Check sheet for the modelled part. Datum: model origin and axes. Units: mm. A direction names the side the tool comes from. Round coordinates to 2 decimals unless told otherwise and drop trailing zeros. Write each loop counter-clockwise with the first axis right and the second up, starting at its lowest first coordinate (ties: lowest second). Pieces come first, ordered by that corner, then holes. Notation, with made-up numbers: M 2,31 L 47,31 A27 ccw 47,47 Z; hole C 74,-23.75 d3. An arc over 180 degrees is marked long. One line per item, written item: value.
from build123d import *

# Parameters (mm, degrees)
F0_W     = 95.25
F0_H     = 304.8
F0_W_2   = 69.85
F0_H_2   = 292.1
F1_DEPTH = 69.85
F2_DEPTH = 6.35
F3_W     = 69.85
F3_H     = 76.2
F4_DEPTH = 6.35
F6_DEPTH = 450.85


with BuildPart() as f1:
    # F0 (on Top) → F1 (new body)
    with BuildSketch(Plane.XY):
        Rectangle(F0_W, F0_H)
        Rectangle(F0_W_2, F0_H_2, mode=Mode.SUBTRACT)
    extrude(amount=F1_DEPTH)

    # F0 (on Top) → F2 (join)
    with BuildSketch(Plane.XY):
        Rectangle(F0_W, F0_H)
        Rectangle(F0_W_2, F0_H_2, mode=Mode.SUBTRACT)
        Rectangle(F0_W_2, F0_H_2)
    extrude(amount=-F2_DEPTH)

    # F3 (on face) → F4 (cut)
    with BuildSketch(Plane(origin=(0, 0, -6.35), x_dir=(1, 0, 0), z_dir=(0, 0, -1))):
        with Locations((0, -107.95)):
            Rectangle(F3_W, F3_H)
    extrude(amount=-F4_DEPTH, mode=Mode.SUBTRACT)

    # F5 (on face) → F6 (join)
    with BuildSketch(Plane(origin=(0, 0, -6.35), x_dir=(1, 0, 0), z_dir=(0, 0, -1))):
        Polygon((-47.625, -152.4), (47.625, -152.4), (47.625, -95.25), (34.925, -95.25), (34.925, -146.05), (-34.925, -146.05), (-34.925, -95.25), (-47.625, -95.25), align=None)
    extrude(amount=F6_DEPTH)


solid = f1.part
Q1. Access from +Z, -Z, +X, -X, +Y, -Y to the whole of each face (thin tool, end or side, straight path). Record for faces 1 (the flat face through (34.925, 97, -75)), 2 (the flat face through (-41, 95.25, -229)), 3 (the flat face through (-1, -152.4, 32)).
Completed:
face 1: +Z
face 2: -Z, +X, -X, -Y
face 3: +Z, -Z, +X, -X, -Y
Q2. Sectioned sample at A-A on x = 9. Enter the section's corners in (y, z).
Completed:
outline: M -152.4,-6.35 L 69.85,-6.35 L 69.85,0 L -146.05,0 L -146.05,69.85 L -152.4,69.85 Z; M 146.05,-457.2 L 152.4,-457.2 L 152.4,69.85 L 146.05,69.85 Z
Q3. Depth check by flat-ended pin: P1, Ø3, axis at x = -22.5, y = -94, coming from the +Z side; P2, Ø4, axis at x = -41.5, z = -344, coming from the -Y side; P3, Ø2, axis at x = -19, y = 14, coming from the -Z side. Enter the tip coordinate at first touch or a pass-through.
Completed:
P1: z = 0
P2: y = 95.25
P3: z = -6.35
Q4. Scan lines: line 1 (X direction, y = -36.5, z = 48.5) (3 decimals); line 2 (Y direction, x = -6.5, z = 6.5); line 3 (Y direction, x = 36.5, z = -415.5). Record each from-to range of solid material in increasing order. Write a range as [from, to].
Completed:
line 1: [-47.625, -34.925], [34.925, 47.625]
line 2: [-152.4, -146.05], [146.05, 152.4]
line 3: [95.25, 152.4]
Q5. Sectioned sample at D-D on z = -70. Enter the section's corners in (x, y) (3 decimals), and give its area (3 significant figures).
Completed:
outline: M -47.625,95.25 L -34.925,95.25 L -34.925,146.05 L 34.925,146.05 L 34.925,95.25 L 47.625,95.25 L 47.625,152.4 L -47.625,152.4 Z
area: 1,900 mm^2
Q6. Sectioned sample at C-C on z = 32. Enter the section's corners in (x, y) (3 decimals).
Completed:
outline: M -47.625,-152.4 L 47.625,-152.4 L 47.625,152.4 L -47.625,152.4 Z; hole M -34.925,-146.05 L 34.925,-146.05 L 34.925,146.05 L -34.925,146.05 Z
Q7. Sectioned sample at B-B on y = 78.5. Enter the section's corners in (x, z) (3 decimals), and give its area (3 significant figures).
Completed:
outline: M -47.625,-6.35 L -34.925,-6.35 L -34.925,69.85 L -47.625,69.85 Z; M 34.925,-6.35 L 47.625,-6.35 L 47.625,69.85 L 34.925,69.85 Z
area: 1,940 mm^2
